```python
from build123d import *

# Parameters (mm, degrees)
SKETCH_1_R               = 1.6
EXTRUDE_1_DEPTH          = 3
SKETCH_2_W               = 7
SKETCH_2_H               = 14
EXTRUDE_2_DEPTH          = 10
CUT_EXTRUDE_1_DEPTH      = 115.456323547
CUT_EXTRUDE_1_DEPTH_BACK = 115.456323547
SKETCH_4_R               = 1.6
FILLET_1_R               = 2
CUT_EXTRUDE_2_DEPTH      = 3
CUT_EXTRUDE_START        = -3
CUT_EXTRUDE_3_DEPTH      = 3


with BuildPart() as part:
    # 草图1 → 凸台-拉伸1 (new body)
    with BuildSketch(Plane.XY):
        with BuildLine():
            Line((-10, 103.998111102), (-10, 95.043808085))
            ThreePointArc((-10, 95.043808085), (-11.2, 90), (-10, 84.956191915))
            Line((-10, 84.956191915), (-10, 75))
            Line((-10, 75), (-17, 75))
            ThreePointArc((-17, 75), (-19.121320344, 75.878679656), (-20, 78))
            Line((-20, 78), (-20, 104))
            ThreePointArc((-20, 104), (-19.121320344, 106.121320344), (-17, 107))
            Line((-17, 107), (17, 107))
            ThreePointArc((17, 107), (19.121320344, 106.121320344), (20, 104))
            Line((20, 104), (20, 78))
            ThreePointArc((20, 78), (19.121320344, 75.878679656), (17, 75))
            Line((17, 75), (10, 75))
            Line((10, 75), (10, 84.956191915))
            ThreePointArc((10, 84.956191915), (11.2, 90), (10, 95.043808085))
            Line((10, 95.043808085), (10, 103.998111102))
            Line((10, 103.998111102), (-10, 103.998111102))
        make_face()
        with Locations((-13, 102)):
            Circle(SKETCH_1_R, mode=Mode.SUBTRACT)
        with Locations((-13, 78)):
            Circle(SKETCH_1_R, mode=Mode.SUBTRACT)
        with Locations(Location((13, 102, 0), (0, 0, 180))):
            Circle(SKETCH_1_R, mode=Mode.SUBTRACT)
        with Locations(Location((13, 78, 0), (0, 0, 180))):
            Circle(SKETCH_1_R, mode=Mode.SUBTRACT)
    extrude(amount=EXTRUDE_1_DEPTH)

    # 草图2 → 凸台-拉伸2 (add)
    with BuildSketch(Plane.XY.offset(3)):
        with Locations((-15, 90)):
            Rectangle(SKETCH_2_W, SKETCH_2_H)
        with Locations((15, 90)):
            Rectangle(SKETCH_2_W, SKETCH_2_H)
    extrude(amount=EXTRUDE_2_DEPTH)

    # 草图4 → 切除-拉伸1 (cut, two sides: drawn at the far end of the back side and taken through both)
    with BuildSketch(Plane.ZY.offset(18.5).offset(-CUT_EXTRUDE_1_DEPTH_BACK)):
        with Locations((9.5, 93)):
            Circle(SKETCH_4_R)
        with Locations((9.5, 87)):
            Circle(SKETCH_4_R)
    extrude(amount=CUT_EXTRUDE_1_DEPTH + CUT_EXTRUDE_1_DEPTH_BACK, mode=Mode.SUBTRACT)

    # 圆角1
    fillet_1_edges = [part.edges().sort_by_distance(p)[0] for p in [
        (-10, 75, 1.5),
        (10, 75, 1.5),
        (10, 103.998111102, 1.5),
        (-10, 103.998111102, 1.5),
    ]]
    fillet(fillet_1_edges, radius=FILLET_1_R)

    # 草图5 → 切除-拉伸2 (cut)
    with BuildSketch(Plane.ZY.offset(-11.5)):
        with BuildLine():
            Line((12.5, 93), (12.5, 87))
            ThreePointArc((12.5, 87), (9.5, 84), (6.5, 87))
            Line((6.5, 87), (6.5, 93))
            ThreePointArc((6.5, 93), (9.5, 96), (12.5, 93))
        make_face()
    extrude(amount=-CUT_EXTRUDE_2_DEPTH, mode=Mode.SUBTRACT)

    # 草图6 → 切除-拉伸3 (cut)
    with BuildSketch(Plane(origin=(-11.5, 0, 0), x_dir=(0, 0, -1), z_dir=(1, 0, 0)).offset(CUT_EXTRUDE_START)):
        with BuildLine():
            Line((-6.5, 93), (-6.5, 87))
            ThreePointArc((-6.5, 87), (-9.5, 84), (-12.5, 87))
            Line((-12.5, 87), (-12.5, 93))
            ThreePointArc((-12.5, 93), (-9.5, 96), (-6.5, 93))
        make_face()
    extrude(amount=CUT_EXTRUDE_3_DEPTH, mode=Mode.SUBTRACT)


solid = part.part
```
Check sheet for the modelled part. Datum: model origin and axes. Units: mm. A direction names the side the tool comes from. Coordinates: 2 decimals unless noted, no trailing zeros. Write each loop counter-clockwise with the first axis right and the second up, starting at its lowest first coordinate (ties: lowest second). Pieces come first, ordered by that corner, then holes. Notation, with made-up numbers: M 61.5,-11 L 92.5,-11 A6 cw 92.5,-2 Z; hole C 60.5,44.5 d3. An arc over 180 degrees is marked long. Use one line per item in the form item = value.
Item 1: Release check for a two-part mould opening along Y. For faces 4 (the face through (-15, 97, 8)), 5 (the face through (-13, 90, 6.5)), 6 (the face through (20, 91, 1)), 7 (the face through (-16.472, 88.586, 9.292)) record: pulls with the +Y half, pulls with the -Y half, needs draft (parallel to the pull), parting line crosses it, or undercut.
Answer below:
face_4 = pulls with the +Y half
face_5 = undercut
face_6 = needs draft
face_7 = undercut
Item 2: Sectioned sample at A-A, the plane x = -13. Record the cut outline in (y, z), and give its area (3 significant figures).
Answer below:
outline = M 75,0 L 76.4,0 L 76.4,3 L 75,3 Z; M 79.6,0 L 100.4,0 L 100.4,3 L 97,3 L 97,13 L 83,13 L 83,3 L 79.6,3 Z; M 103.6,0 L 107,0 L 107,3 L 103.6,3 Z; hole M 87,6.5 L 93,6.5 A3 ccw 93,12.5 L 87,12.5 A3 ccw Z
area = 153 mm^2
Item 3: Sectioned sample at D-D, the plane y = 98.5. Record the cut outline in (x, z).
Answer below:
outline = M -20,0 L -10,0 L -10,3 L -20,3 Z; M 10,0 L 20,0 L 20,3 L 10,3 Z
Item 4: Set-up check for faces 1 (the face through (13, 90, 6.5)), 2 (the face through (-10.57, 75.6, 1.52)), 3 (the face through (-20, 91, 1)): record each of +Z, -Z, +X, -X, +Y, -Y from which the full face is reachable in a straight line by a thin tool's end or side.
Answer below:
face_1 = none
face_2 = +Z, -Z, -Y
face_3 = +Z, -Z, -X, +Y, -Y
Item 5: Sectioned sample at B-B, the plane z = 5. Record the cut outline in (x, y).
Answer below:
outline = M -18.5,83 L -11.5,83 L -11.5,97 L -18.5,97 Z; M 11.5,83 L 18.5,83 L 18.5,97 L 11.5,97 Z
Item 6: Material ranges on L1, parallel to X at y = 102, z = 2.45; L2, parallel to Y at x = -17, z = 9.5; L3, parallel to Y at x = 13, z = 1.8, recorded low to high. Write a range as from..to.
Answer below:
L1 = -20..-14.6, -11.4..-10, 10..11.4, 14.6..20
L2 = 83..85.4, 88.6..91.4, 94.6..97
L3 = 75..76.4, 79.6..100.4, 103.6..107
Item 7: Sectioned sample at C-C, the plane z = 9.5. State how many separate pieces and enclosed holes the cut face has, and give its area (3 significant figures).
Answer below:
separate_pieces = 6
enclosed_holes = 0
area = 72.8 mm^2
Item 8: Gauge pin test, flat ends, axial feed: pin 1 Ø5 at (y, z) = (89.5, 8.5) entering from +X; pin 2 Ø1.5 at (x, z) = (-14, 8.5) entering from +Y; pin 3 Ø2 at (x, y) = (-12.5, 102.5) entering from +Z. Record the tip position at first contact, or that the pin passes through.
Answer below:
pin_1 = 18.5
pin_2 = 97
pin_3 = 3
